CAD build for the part. Positions are in the model's coordinates, mm. A direction names the side the tool comes from. Round coordinates to 2 decimals unless told otherwise and drop trailing zeros. Write each loop counter-clockwise with the first axis right and the second up, starting at its lowest first coordinate (ties: lowest second). Pieces come first, ordered by that corner, then holes. Notation, with made-up numbers: (13.25, -36) - (71.25, -36) arc R23 cw to (71.25, -13) - close; hole circle Ø6 at (42, 55). An arc over 180 degrees is marked (long way). Put each result on its own line as item: value. Start each with the question number.
Item 1: Mould opens along X. For faces 4 (the flat face through (24, 20, 0)), 5 (the flat face through (30, 8, 0)), 6 (the flat face through (59, 13, 0)) say: released by +X, released by -X, zero draft, split by the parting line, or undercut.
Item 2: Pin check, flat tips, straight feed: pin 1 Ø1.5 at (y, z) = (7, -5.5) entering from -X; pin 2 Ø12 at (x, z) = (8, 8) entering from -Y. Stop position of each tip, or through.
Item 3: Drill centre lines: line 1 (X direction, y = 8, z = 2); line 2 (Y direction, x = 1, z = 1.5). Where is each one in solid material? Low to high. Write a range as from..to.
Item 4: Cut at C-C (x = 12). Give the cut face in (y, z), and give its area (3 significant figures).
Item 5: 3-axis set-ups, long thin cutter, end or side, ignore diameter. For faces 1 (the flat face through (20, 7, 0)), 2 (the flat face through (40, 10, 0)), 3 (the flat face through (24, 14, 12.5)): which of +Z, -Z, +X, -X, +Y, -Y reach the whole face in a straight line?
Item 6: Cut at B-B (z = 2). Give the cut face in (x, y).
Item 7: Cut at A-A (y = 8.25). Give the cut face in (x, z).
Autodesk Inventor part; units mm, degrees
ref_plane "YZ Plane" through (0, 0, 0) normal (1, 0, 0) x (0, 1, 0)
ref_plane "XZ Plane" through (0, 0, 0) normal (0, 1, 0) x (-1, 0, 0)
ref_plane "XY Plane" through (0, 0, 0) normal (0, 0, 1) x (1, 0, 0)
sketch "Sketch1" plane through (0, 0, 0) normal (0, 0, 1) x (1, 0, 0)
  line L0 (-10, 10) -> (-10, 20)
  line L1 (-10, 20) -> (59, 20)
  line L2 (59, 20) -> (59, 5)
  line L3 (59, 5) -> (49, 5)
  line L4 (49, 5) -> (49, 10)
  line L5 (49, 10) -> (30, 10)
  line L6 (30, 10) -> (30, 5)
  line L7 (30, 5) -> (20, 5)
  line L8 (20, 5) -> (20, 10)
  line L9 (20, 10) -> (-10, 10)
  point P0 (0, 0)
  point P1 (0, 0)
  dimension "d0" = 19
  dimension "d1" = 10
  dimension "d2" = 10
  dimension "d3" = 30
  dimension "d4" = 10
  dimension "d5" = 5
  dimension "d6" = 59
  dimension "d7" = 10
  dimension "d8" = 10
  dimension "d9" = 59
extrude "Extrusion1" add sketch "Sketch1" along normal mid plane 25
properties part number "Load cell holder 3D print"
Output values:
1. face 4: zero draft
1. face 5: undercut
1. face 6: released by +X
2. pin 1: x = 20
2. pin 2: y = 10
3. line 1: 20..30, 49..59
3. line 2: 10..20
4. outline: (10, -12.5) - (20, -12.5) - (20, 12.5) - (10, 12.5) - close
4. area: 250 mm2
5. face 1: +Z, -Z, -X, -Y
5. face 2: +Z, -Z, -Y
5. face 3: +Z, +X, -X, +Y, -Y
6. outline: (-10, 10) - (20, 10) - (20, 5) - (30, 5) - (30, 10) - (49, 10) - (49, 5) - (59, 5) - (59, 20) - (-10, 20) - close
7. outline: (20, -12.5) - (30, -12.5) - (30, 12.5) - (20, 12.5) - close; (49, -12.5) - (59, -12.5) - (59, 12.5) - (49, 12.5) - close
